from build123d import *

# Parameters (mm, degrees)
SKETCH1_R           = 9.779
BOSS_EXTRUDE1_DEPTH = 4.953
SKETCH2_R           = 1.905
BOSS_EXTRUDE2_DEPTH = 0.508
SKETCH3_R           = 6.578574276
SKETCH3_R_2         = 4.119665811
CUT_EXTRUDE1_DEPTH  = 0.508
SKETCH4_W           = 6.183927722
SKETCH4_H           = 2.240204311
BOSS_EXTRUDE3_DEPTH = 35.56
SKETCH5_W           = 2.60391419
SKETCH5_H           = 6.183927722
BOSS_EXTRUDE4_DEPTH = 12.7


with BuildPart() as part:
    # Sketch1 → Boss-Extrude1 (new body)
    with BuildSketch(Plane(origin=(0, 0, 0), x_dir=(1, 0, 0), z_dir=(0, 1, 0))):
        Circle(SKETCH1_R)
    extrude(amount=BOSS_EXTRUDE1_DEPTH)

    # Sketch2 → Boss-Extrude2 (add)
    with BuildSketch(Plane(origin=(0, 4.953, 0), x_dir=(1, 0, 0), z_dir=(0, 1, 0))):
        Circle(SKETCH2_R)
    extrude(amount=BOSS_EXTRUDE2_DEPTH)

    # Sketch3 → Cut-Extrude1 (cut)
    with BuildSketch(Plane(origin=(0, 4.953, 0), x_dir=(1, 0, 0), z_dir=(0, 1, 0))):
        Circle(SKETCH3_R)
        Circle(SKETCH3_R_2, mode=Mode.SUBTRACT)
    extrude(amount=-CUT_EXTRUDE1_DEPTH, mode=Mode.SUBTRACT)

    # Sketch4 → Boss-Extrude3 (add)
    with BuildSketch(Plane(origin=(0, 0, 0), x_dir=(0, 0, -1), z_dir=(1, 0, 0))):
        with Locations((0, 1.120102156)):
            Rectangle(SKETCH4_W, SKETCH4_H)
    extrude(amount=BOSS_EXTRUDE3_DEPTH)

    # Sketch5 → Boss-Extrude4 (add)
    with BuildSketch(Plane.XZ):
        with Locations((34.258042905, 0)):
            Rectangle(SKETCH5_W, SKETCH5_H)
    extrude(amount=BOSS_EXTRUDE4_DEPTH)


solid = part.part
CAD build for the part. Positions are in the model's coordinates, mm. A direction names the side the tool comes from. Coordinates: 2 decimals unless noted, no trailing zeros. Write each loop counter-clockwise with the first axis right and the second up, starting at its lowest first coordinate (ties: lowest second). Pieces come first, ordered by that corner, then holes. Notation, with made-up numbers: M 8.5,7.25 L 39.5,7.25 A29 ccw 39.5,30.25 Z; hole C 55,-5 d4. An arc over 180 degrees is marked long. Answer as a JSON object with one key per item and string values. Group by question number.
1) Saw through at C-C (y = 1.75). Write the cut outline in (x, z), plus the area to 3 significant figures.
2) Saw through at D-D (z = 2.5). Write the cut outline in (x, y) (3 decimals).
3) Tool access for faces 1 (the face through (27, 1, -3.092)), 2 (the face through (32.956, -6, 0)), 3 (the face through (27, 1, 3.092)), 4 (the face through (2, 4.953, 1)): list every direction of +Z, -Z, +X, -X, +Y, -Y with a clear straight run to the whole face (end or side of a thin tool).
4) Saw through at B-B (x = 0). Write the cut outline in (y, z) (3 decimals), plus the area to 3 significant figures.
5) Pin check, flat tips, straight feed: pin 1 Ø2 at (x, z) = (4, 7) entering from +Y; pin 2 Ø4 at (y, z) = (3.5, -4) entering from -X; pin 3 Ø10.5 at (x, z) = (0, 0) entering from -Y; pin 4 Ø4.5 at (x, y) = (18, -2.5) entering from +Z. Stop position of each tip, or through.
6) Wall check: line 1 (X direction, y = 4.7, z = 0); line 2 (X direction, y = -1.5, z = 2). Give the ranges that are in metal, low to high. Write a range as from..to.
7) Mould opens along Z. For faces 5 (the face through (7, 0, 0)), 6 (the face through (-7.76, 2.44, 5.95)), 7 (the face through (4.3, 4.445, -0.1)), 8 (the face through (-1.43, 4.7, 6.42)) say: +Z half, -Z half, draft (parallel to the pull), parting line (faces both ways), or undercut.
8) Saw through at A-A (z = 0). Write the cut outline in (x, y) (3 decimals), plus the area to 3 significant figures.
Values follow:
{
 "1": {"outline": "M 9.28,-3.09 L 35.56,-3.09 L 35.56,3.09 L 9.28,3.09 A9.78 ccw long Z", "area": "461 mm2"},
 "2": {"outline": "M -9.454,0 L 32.956,0 L 32.956,-12.7 L 35.56,-12.7 L 35.56,2.24 L 9.454,2.24 L 9.454,4.953 L 6.085,4.953 L 6.085,4.445 L 3.274,4.445 L 3.274,4.953 L -3.274,4.953 L -3.274,4.445 L -6.085,4.445 L -6.085,4.953 L -9.454,4.953 Z"},
 "3": {"face 1": "-Z, +X, +Y, -Y", "face 2": "+Z, -Z, -X, -Y", "face 3": "+Z, +X, +Y, -Y", "face 4": "+Y"},
 "4": {"outline": "M 0,-9.779 L 4.953,-9.779 L 4.953,-6.579 L 4.445,-6.579 L 4.445,-4.12 L 4.953,-4.12 L 4.953,-1.905 L 5.461,-1.905 L 5.461,1.905 L 4.953,1.905 L 4.953,4.12 L 4.445,4.12 L 4.445,6.579 L 4.953,6.579 L 4.953,9.779 L 0,9.779 Z", "area": "96.3 mm2"},
 "5": {"pin 1": "stops at y = 4.95", "pin 2": "stops at x = -9.57", "pin 3": "stops at y = 0", "pin 4": "passes through"},
 "6": {"line 1": "x = -9.78..-6.58, -4.12..4.12, 6.58..9.78", "line 2": "x = 32.96..35.56"},
 "7": {"face 5": "draft", "face 6": "parting line", "face 7": "undercut", "face 8": "undercut"},
 "8": {"outline": "M -9.779,0 L 32.956,0 L 32.956,-12.7 L 35.56,-12.7 L 35.56,2.24 L 9.779,2.24 L 9.779,4.953 L 6.579,4.953 L 6.579,4.445 L 4.12,4.445 L 4.12,4.953 L 1.905,4.953 L 1.905,5.461 L -1.905,5.461 L -1.905,4.953 L -4.12,4.953 L -4.12,4.445 L -6.579,4.445 L -6.579,4.953 L -9.779,4.953 Z", "area": "187 mm2"}
}
